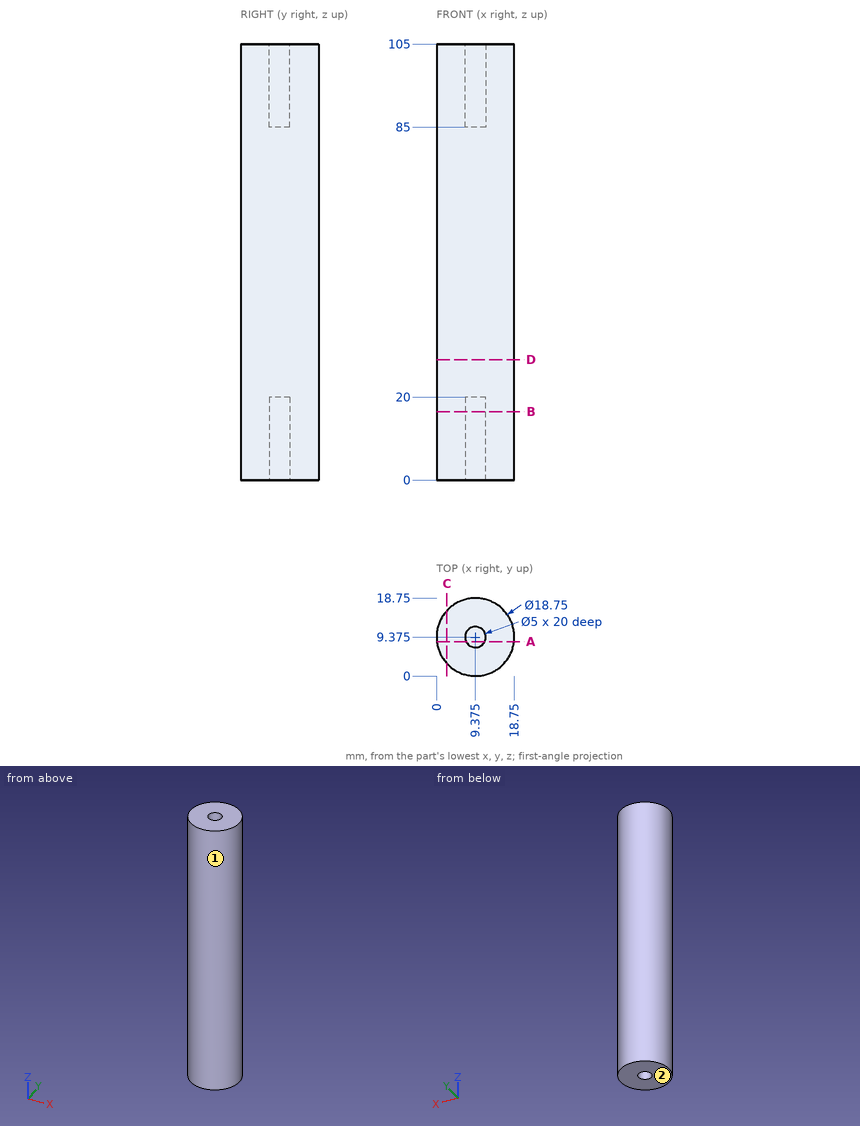
The figure shows three views and two pictorial views of one solid part (mm, origin at its lowest corner). Answer the questions. Round coordinates to 2 decimals unless told otherwise and drop trailing zeros. Write each loop counter-clockwise with the first axis right and the second up, starting at its lowest first coordinate (ties: lowest second). Pieces come first, ordered by that corner, then holes. Notation, with made-up numbers: M 23,82.5 L 32,82.5 A30 ccw 32,121.5 Z; hole C -25.75,-8.75 d3. An arc over 180 degrees is marked long. Use a Markdown table: item, result.
1) The part is cut by section C-C (x = 2.5). Write down the section's boundary in (y, z).
Answers follow:
| item | result |
|---|---|
| outline | M 3,0 L 15.75,0 L 15.75,105 L 3,105 Z |
2) Flat-ended cylindrical pins translate along their axes: pin 1 (1.5 mm diameter, centred on x = 9, y = 9, fed in from -Z); pin 2 (10 mm diameter, centred on x = 3.5, z = 23.5, fed in from -Y); pin 3 (4 mm diameter, centred on x = 5.5, z = 50, fed in from +Y). Find the tip coordinate at first contact, or state that the pin passes through.
Answers follow:
| item | result |
|---|---|
| pin 1 | stops at z = 20 |
| pin 2 | stops at y = 0.04 |
| pin 3 | stops at y = 18.56 |
3) The part is cut by section B-B (z = 16.5). Write down the section's boundary in (x, y) (3 decimals), plus the area to 3 significant figures.
Answers follow:
| item | result |
|---|---|
| outline | C 9.375,9.375 d18.75; hole C 9.375,9.375 d5 |
| area | 256 mm2 |
4) The part is cut by section D-D (z = 29). Write down the section's boundary in (x, y) (3 decimals).
Answers follow:
| item | result |
|---|---|
| outline | C 9.375,9.375 d18.75 |
5) For a pull along Y with two mould halves and no side action, classify the marked faces 1 and 2 as pulls with the +Y half, pulls with the -Y half, needs draft (parallel to the pull), parting line crosses it, or undercut.
Answers follow:
| item | result |
|---|---|
| face 1 | parting line crosses it |
| face 2 | needs draft |
6) Straight lines are drawn through the part: line 1 along X through (y, z) = (10, 92); line 2 along Y through (x, z) = (11, 16); line 3 along Y through (x, z) = (8, 85.5). For each, find the intervals that lie inside material, in ascending order. Write a range as [from, to].
Answers follow:
| item | result |
|---|---|
| line 1 | x = [0.02, 6.95], [11.8, 18.73] |
| line 2 | y = [0.14, 7.48], [11.27, 18.61] |
| line 3 | y = [0.1, 7.29], [11.46, 18.65] |
7) The part is cut by section A-A (y = 8.25). Write down the section's boundary in (x, z).
Answers follow:
| item | result |
|---|---|
| outline | M 0.07,0 L 7.14,0 L 7.14,20 L 11.61,20 L 11.61,0 L 18.68,0 L 18.68,105 L 11.61,105 L 11.61,85 L 7.14,85 L 7.14,105 L 0.07,105 Z |
